For this review, take the finished solid that the model builds, in its own axes (mm). A direction names the side the tool comes from. Coordinates: 2 decimals unless noted, no trailing zeros. Loops run counter-clockwise (first coordinate to the right, second up) from the corner with the lowest first, then second, coordinate; pieces in that order, holes last. Notation, with made-up numbers: M 65.5,52 L 76.5,52 A10 ccw 76.5,66 Z; hole C -12,-38.5 d1. An arc over 180 degrees is marked long. Use one line per item in the form item = value.
```python
from build123d import *

# Parameters (mm, degrees)
ESQUISSE1_W             = 15.8
ESQUISSE1_H             = 62
BOSS_EXTRU_1_DEPTH      = 1.8
ESQUISSE2_W             = 13.8
ESQUISSE2_H             = 61
BOSS_EXTRU_2_DEPTH      = 1
CONG_1_R                = 1.5
ESQUISSE3_W             = 15.8
ESQUISSE3_H             = 1
ENL_V_MAT_EXTRU_1_DEPTH = 10


with BuildPart() as part:
    # Esquisse1 → Boss.-Extru.1 (new body)
    with BuildSketch(Plane(origin=(0, 0, 0), x_dir=(1, 0, 0), z_dir=(0, 1, 0))):
        with Locations((7.9, 31)):
            Rectangle(ESQUISSE1_W, ESQUISSE1_H)
    extrude(amount=BOSS_EXTRU_1_DEPTH)

    # Esquisse2 → Boss.-Extru.2 (add)
    with BuildSketch(Plane(origin=(0, 1.8, 0), x_dir=(1, 0, 0), z_dir=(0, 1, 0))):
        with Locations((7.9, 31.5)):
            Rectangle(ESQUISSE2_W, ESQUISSE2_H)
    extrude(amount=BOSS_EXTRU_2_DEPTH)

    # Congé1
    cong_1_edges = [part.edges().sort_by_distance(p)[0] for p in [
        (7.9, 2.8, -62),
    ]]
    fillet(cong_1_edges, radius=CONG_1_R)

    # Esquisse3 → Enlèv. mat.-Extru.1 (cut)
    with BuildSketch(Plane(origin=(0, 2.8, 0), x_dir=(1, 0, 0), z_dir=(0, 1, 0))):
        with Locations((7.9, 0.5)):
            Rectangle(ESQUISSE3_W, ESQUISSE3_H)
    extrude(amount=-ENL_V_MAT_EXTRU_1_DEPTH, mode=Mode.SUBTRACT)


solid = part.part
```
1. Consider section B-B on y = 2.25. Write out the cut boundary in (x, z).
Computed values:
outline = M 1,-61.66 L 14.8,-61.66 L 14.8,-1 L 1,-1 Z
2. Wall thickness on line 1 along X through (y, z) = (2.45, -13); line 2 along Z through (x, y) = (6.5, 2.2); line 3 along Z through (x, y) = (8.5, 1.85): over which ranges is each line inside the solid? List them lowest first. Write a range as from..to.
Computed values:
line_1 = 1..14.8
line_2 = -61.7..-1
line_3 = -61.9..-1
3. For pin 1 Ø1.1 at (y, z) = (2.5, -33.5) entering from +X; pin 2 Ø0.8 at (x, z) = (0.5, -39) entering from +Y, all flat-tipped, find the tip position at first contact; note any pin that passes through.
Computed values:
pin_1 = 14.8
pin_2 = 1.8
4. Consider section A-A on z = -18. Write out the cut boundary in (x, y).
Computed values:
outline = M 0,0 L 15.8,0 L 15.8,1.8 L 14.8,1.8 L 14.8,2.8 L 1,2.8 L 1,1.8 L 0,1.8 Z
5. Tool access review of faces 1 (the face through (1, 2, -31)), 2 (the face through (8, 2.8, -31)), 3 (the face through (14.8, 2, -31)): name each direction out of +Z, -Z, +X, -X, +Y, -Y from which nothing blocks a thin tool from reaching the whole face with its end or side.
Computed values:
face_1 = +Z, -Z, -X, +Y
face_2 = +Z, -Z, +X, -X, +Y
face_3 = +Z, -Z, +X, +Y
